Input: part model. Units: mm. Frame: model coordinates. Face numbers are marked on the shaded views. Coordinates: 2 decimals unless noted, no trailing zeros. Loops run counter-clockwise (first coordinate to the right, second up) from the corner with the lowest first, then second, coordinate; pieces in that order, holes last. Notation, with made-up numbers: (-12, 79) -> (11, 79) arc R9 cw to (11, 94) -> close; hole circle Ø4 at (33.25, 9.25). An arc over 180 degrees is marked (long way). Answer as a JSON object with one key per item and string values.
from build123d import *

# Parameters (mm, degrees)
SKETCH1_W           = 84
SKETCH1_H           = 80
BOSS_EXTRUDE1_DEPTH = 2
SKETCH3_W           = 80
SKETCH3_H           = 76
SKETCH3_W_2         = 76
SKETCH3_H_2         = 72
BOSS_EXTRUDE2_DEPTH = 2
FILLET1_R           = 2
FILLET2_R           = 2
FILLET3_R           = 0.5


with BuildPart() as part:
    # Sketch1 → Boss-Extrude1 (new body)
    with BuildSketch(Plane(origin=(0, 0, 0), x_dir=(1, 0, 0), z_dir=(0, 1, 0))):
        with Locations((42, 40)):
            Rectangle(SKETCH1_W, SKETCH1_H)
    extrude(amount=BOSS_EXTRUDE1_DEPTH)

    # Sketch3 → Boss-Extrude2 (add)
    with BuildSketch(Plane(origin=(0, 2, 0), x_dir=(1, 0, 0), z_dir=(0, 1, 0))):
        with Locations((42.1, 40)):
            Rectangle(SKETCH3_W, SKETCH3_H)
        with Locations((42.106134664, 40.19047619)):
            Rectangle(SKETCH3_W_2, SKETCH3_H_2, mode=Mode.SUBTRACT)
    extrude(amount=BOSS_EXTRUDE2_DEPTH)

    # Fillet1
    fillet1_edges = [part.edges().sort_by_distance(p)[0] for p in [
        (0, 1, -80),
        (84, 1, -80),
        (84, 1, 0),
        (0, 1, 0),
    ]]
    fillet(fillet1_edges, radius=FILLET1_R)

    # Fillet2
    fillet2_edges = [part.edges().sort_by_distance(p)[0] for p in [
        (0.585786438, 0, -0.585786438),
        (0.585786438, 0, -79.414213562),
        (83.414213562, 0, -79.414213562),
        (83.414213562, 0, -0.585786438),
        (84, 0, -40),
        (42, 0, -80),
        (0, 0, -40),
        (42, 0, 0),
    ]]
    fillet(fillet2_edges, radius=FILLET2_R - 0.0001)  # a hair under: the kernel refuses the full size

    # Fillet3
    fillet3_edges = [part.edges().sort_by_distance(p)[0] for p in [
        (42.1, 4, -2),
        (82.1, 4, -40),
        (42.1, 4, -78),
        (2.1, 4, -40),
        (42.106134664, 4, -4.19047619),
        (80.106134664, 4, -40.19047619),
        (42.106134664, 4, -76.19047619),
        (4.106134664, 4, -40.19047619),
    ]]
    fillet(fillet3_edges, radius=FILLET3_R)


solid = part.part
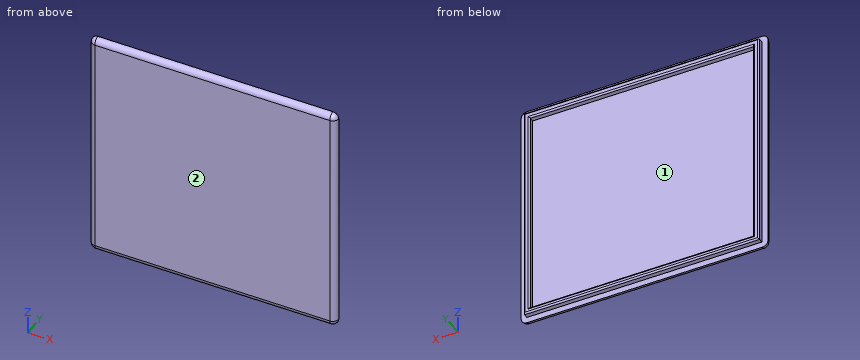
1. Section query A-A (y = 2.65). Return loops of the section in (x, z), plus the area to 3 significant figures.
Reply:
{"outline": "(2.1, -78) -> (82.1, -78) -> (82.1, -2) -> (2.1, -2) -> close; hole (4.11, -76.19) -> (80.11, -76.19) -> (80.11, -4.19) -> (4.11, -4.19) -> close", "area": "608 mm2"}
2. Pin query (flat end, axial travel): P1, Ø0.8, axis at x = 53.5, y = 2.5, coming from the -Z side; P2, Ø3, axis at x = 49, z = -10, coming from the +Y side; P3, Ø1.2, axis at y = 3, z = -30, coming from the -X side. Return the tip coordinate at first contact, or that it passes through.
Reply:
{"P1": "stops at z = -78", "P2": "stops at y = 2", "P3": "stops at x = 2.1"}
3. Mould query, pull axis X, two halves, no side actions, for the marked faces 1 and 2. Classes: pulls with the +X half, pulls with the -X half, needs draft (parallel to the pull), parting line crosses it, or undercut.
Reply:
{"face 1": "undercut", "face 2": "needs draft"}
4. Line query: line 1 along Z through (x, y) = (39.5, 3.6); line 2 along X through (y, z) = (3.45, -32); line 3 along Y through (x, z) = (16, -30.5). Output: solid intervals per line, ascending.
Reply:
{"line 1": "z = -77.99 to -76.2, -4.18 to -2.01", "line 2": "x = 2.1 to 4.11, 80.11 to 82.1", "line 3": "y = 0 to 2"}
